Can you work these out from the model? Positions are in its coordinate system, mm. A direction names the side the tool comes from. Give positions to 0.01 mm unless a question says otherwise; leave off trailing zeros. Order: outer loops, then holes, each group sorted by start corner. A loop starts at its lowest first (then second) coordinate and runs counter-clockwise, first axis right, second up.
```python
from build123d import *

# Parameters (mm, degrees)
BOSS_EXTRUDE1_DEPTH = 40
BOSS_EXTRUDE2_DEPTH = 20
SKETCH2_R           = 5
CUT_EXTRUDE1_DEPTH  = 73.972597597


with BuildPart() as part:
    # Sketch1 → Boss-Extrude1 (new body)
    with BuildSketch(Plane.XY):
        Polygon((0, 10), (0, 0), (50, 0), (50, 18), (40, 18), (40, 8), (25, 8), (25, 18), (6.4, 18), align=None)
    extrude(amount=BOSS_EXTRUDE1_DEPTH)

    # Sketch1_4 → Boss-Extrude2 (add)
    with BuildSketch(Plane.XY):
        Polygon((40, 18), (50, 18), (50, 35), (20, 35), (6.4, 18), (25, 18), (25, 28), (40, 28), align=None)
    extrude(amount=BOSS_EXTRUDE2_DEPTH)

    # Sketch2 → Cut-Extrude1 (cut, through all)
    with BuildSketch(Plane(origin=(0, 35, 0), x_dir=(1, 0, 0), z_dir=(0, 1, 0))):
        with Locations(Location((35, -10, 0), (0, 0, 180))):
            Circle(SKETCH2_R)
    extrude(amount=-CUT_EXTRUDE1_DEPTH, mode=Mode.SUBTRACT)


solid = part.part
```
1) Which directions (+Z, -Z, +X, -X, +Y, -Y) give clear straight access to the entire face, cutting with the end or side of a thin tool? Please do faces 1 (the face through (40, 16, 15)), 2 (the face through (16, 18, 30)), 3 (the face through (25, 0, 20)).
2) We'd pull the mould along Z, two halves only. Please class faces 4 (the face through (24.7, 17.7, 0)), 5 (the face through (24.7, 9.1, 40)), 6 (the face through (40, 32, 10)), 7 (the face through (29, 28, 10)): +Z half, -Z half, draft (parallel to the pull), parting line (faces both ways), or undercut.
3) Suppose I cut it at A-A (y = 23). Please give me the cut outline in (x, z), and give its area (3 significant figures).
4) If I drill on line 1 (Z direction, x = 35, y = 5); line 2 (X direction, y = 5, z = 10); line 3 (Z direction, x = 35, y = 32.25), over which ranges is the centre line in solid material (lowest first)?
5) Suppose I cut it at B-B (z = 14). Please give me the cut outline in (x, y).
6) Suppose I cut it at D-D (y = 6). Please give me the cut outline in (x, z), and give its area (3 significant figures).
7) Suppose I cut it at C-C (x = 35). Please give me the cut outline in (y, z), and give its area (3 significant figures).
8) I'm going to push flat-ended pins straight in: pin 1 Ø1 at (y, z) = (18.5, 4.5) entering from -X; pin 2 Ø8.5 at (x, y) = (37, 25) entering from +Z; pin 3 Ø1.5 at (x, z) = (15, 22) entering from +Y. Where does each tip first touch, or does it pass through?
Results:
1. face 1: +Z, -Z
1. face 2: +Z, +X, -X, +Y
1. face 3: +Z, -Z, +X, -X, -Y
2. face 4: -Z half
2. face 5: +Z half
2. face 6: undercut
2. face 7: draft
3. outline: (10.4, 0) - (25, 0) - (25, 20) - (10.4, 20) - close; (40, 0) - (50, 0) - (50, 20) - (40, 20) - close
3. area: 492 mm2
4. line 1: z = 0 to 5, 15 to 40
4. line 2: x = 0 to 30, 40 to 50
4. line 3: z = 0 to 5, 15 to 20
5. outline: (0, 0) - (32, 0) - (32, 8) - (25, 8) - (25, 28) - (32, 28) - (32, 35) - (20, 35) - (0, 10) - close; (38, 0) - (50, 0) - (50, 35) - (38, 35) - (38, 28) - (40, 28) - (40, 8) - (38, 8) - close
6. outline: (0, 0) - (50, 0) - (50, 40) - (0, 40) - close; hole circle Ø10 at (35, 10)
6. area: 1,920 mm2
7. outline: (0, 0) - (8, 0) - (8, 5) - (0, 5) - close; (0, 15) - (8, 15) - (8, 40) - (0, 40) - close; (28, 0) - (35, 0) - (35, 5) - (28, 5) - close; (28, 15) - (35, 15) - (35, 20) - (28, 20) - close
7. area: 310 mm2
8. pin 1: stops at x = 6.4
8. pin 2: stops at z = 20
8. pin 3: stops at y = 18
